The drawing under review shows one solid part. Ordinate dimensions are in mm from its lowest x, y, z. Give positions to 0.01 mm unless a question says otherwise; leave off trailing zeros. Loops run counter-clockwise (first coordinate to the right, second up) from the corner with the lowest first, then second, coordinate; pieces in that order, holes last. Notation, with made-up numbers: (49.25, 39) - (75.25, 39) arc R21 cw to (75.25, 75) - close; hole circle Ø9 at (26, 10). An arc over 180 degrees is marked (long way). Write each question's results on one line, items separated by ' | '.
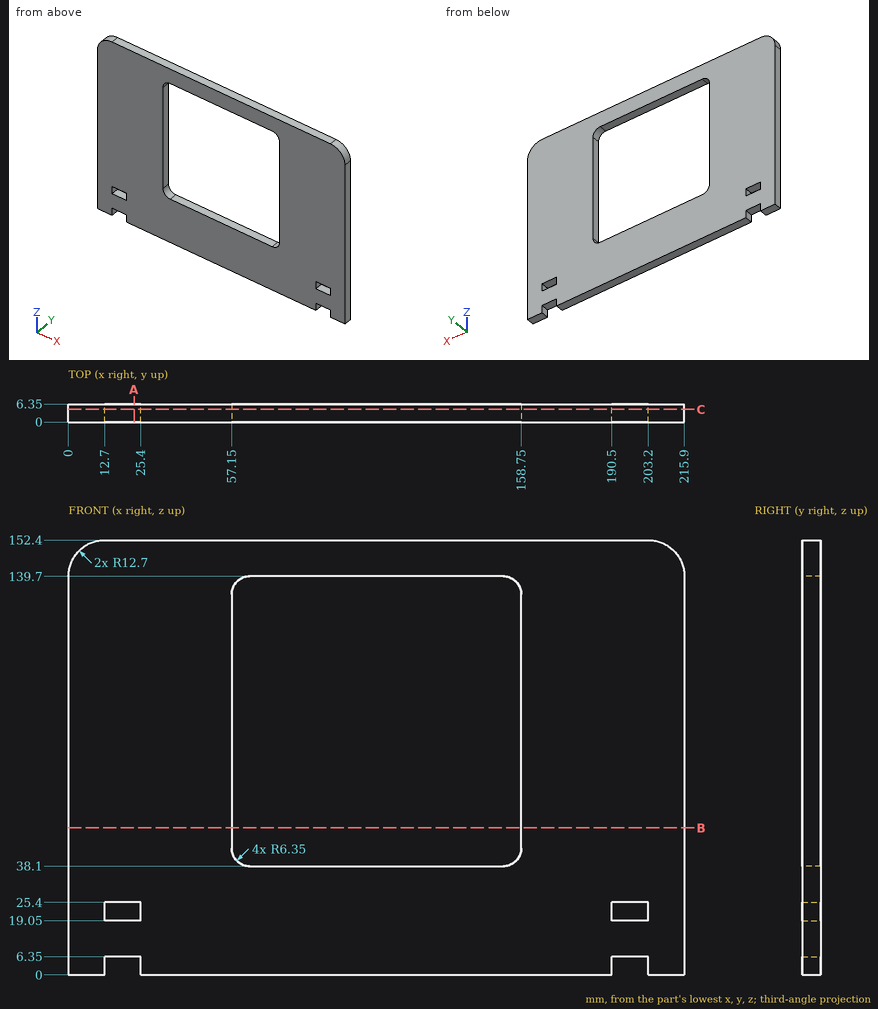
(1) Wall thickness on line 1 along Z through (x, y) = (16, 5); line 2 along X through (y, z) = (2.5, 67.5); line 3 along Z through (x, y) = (114, 3.25): over which ranges is each line inside the solid? List them lowest first. Write a range as from..to.
Answers below:
line 1: 6.35..19.05, 25.4..152.4 | line 2: 0..57.15, 158.75..215.9 | line 3: 0..38.1, 139.7..152.4
(2) Insertion check: P1, Ø1.9, axis at x = 17.5, y = 2, coming from the -Z side; P2, Ø3, axis at y = 2.5, z = 23.5, coming from the -X side. Each pin has a flat end and moves straight along its axis. Give the tip position at first contact, or say it passes through.
Answers below:
P1: z = 6.35 | P2: x = 0
(3) Take a section at A-A on x = 23. Give the boundary of the cut face in (y, z), plus the area to 3 significant figures.
Answers below:
outline: (0, 6.35) - (6.35, 6.35) - (6.35, 19.05) - (0, 19.05) - close; (0, 25.4) - (6.35, 25.4) - (6.35, 152.4) - (0, 152.4) - close | area: 887 mm2
(4) Take a section at C-C on y = 4.5. Count the separate pieces of the cut face and the enclosed holes in it, plus the area to 3 significant figures.
Answers below:
separate pieces: 1 | enclosed holes: 3 | area: 22,200 mm2
(5) Take a section at B-B on z = 51.5. Give the boundary of the cut face in (x, y), plus the area to 3 significant figures.
Answers below:
outline: (0, 0) - (57.15, 0) - (57.15, 6.35) - (0, 6.35) - close; (158.75, 0) - (215.9, 0) - (215.9, 6.35) - (158.75, 6.35) - close | area: 726 mm2
